Here's how the part is built. I have some questions about the finished solid (model axes, mm). Face numbers are marked on the shaded views. A direction names the side the tool comes from. Round coordinates to 2 decimals unless told otherwise and drop trailing zeros. Order: outer loops, then holes, each group sorted by start corner. A loop starts at its lowest first (then second) coordinate and runs counter-clockwise, first axis right, second up. Notation, with made-up numbers: (84, 31.25) - (113, 31.25) arc R19 cw to (113, 51.25) - close; hole circle Ø5 at (8, 25). An arc over 180 degrees is marked (long way). One line per item, written item: value.
from build123d import *

# Parameters (mm, degrees)
SCALE1_SCALE = 1.70603675


with BuildPart() as part:
    # Esquisse1 → Révolution1 (revolve)
    with BuildSketch(Plane.XY, mode=Mode.PRIVATE) as r_volution1_sk:
        with BuildLine():
            Line((1.981656821, 8.97797736), (7.823456821, 8.97797736))
            Line((7.823456821, 8.97797736), (4.683813218, 2.298439639))
            ThreePointArc((4.683813218, 2.298439639), (3.207806254, 0.623149289), (1.06377284, 0))
            Line((1.06377284, 0), (0.803456821, 0))
            Line((0.803456821, 0), (-5.036543179, 0))
            Line((-5.036543179, 0), (-15.076543179, 1.81597736))
            Line((-15.076543179, 1.81597736), (-15.076543179, 4.15197736))
            Line((-15.076543179, 4.15197736), (-2.000513414, 4.15197736))
            ThreePointArc((-2.000513414, 4.15197736), (-1.65849327, 4.212284739), (-1.357725804, 4.385932917))
            Line((-1.357725804, 4.385932917), (-0.12815557, 5.417664847))
            ThreePointArc((-0.12815557, 5.417664847), (0.135364608, 5.761091028), (0.229056821, 6.18370929))
            Line((0.229056821, 6.18370929), (0.229056821, 7.34597736))
            Line((0.229056821, 7.34597736), (1.981656821, 7.34597736))
            Line((1.981656821, 7.34597736), (1.981656821, 8.97797736))
        make_face()
    revolve(r_volution1_sk.sketch.rotate(Axis((-19.476947674, -3.82202264, 0), (1, 0, 0)), 90), axis=Axis((-19.476947674, -3.82202264, 0), (1, 0, 0)))


with BuildPart() as part_1:
    # Scale1: scaled about (-1.246951402, -3.82202264, 0)
    add(part.part.scale(SCALE1_SCALE).moved(Location((0.880393515, 2.698488443, 0))))


solid = part_1.part
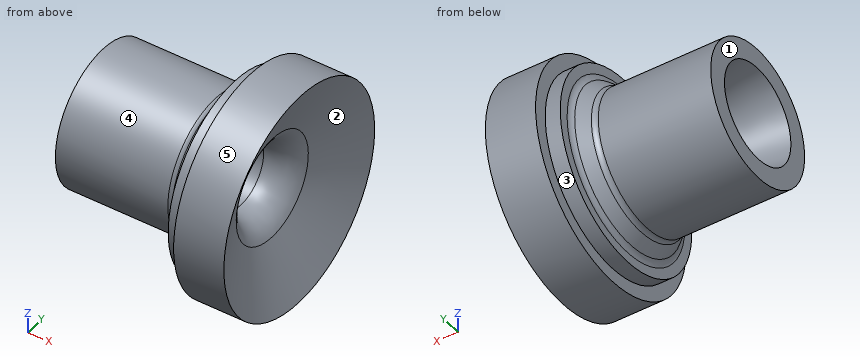
Q1. Which directions (+Z, -Z, +X, -X, +Y, -Y) give clear straight access to the entire face, cutting with the end or side of a thin tool? Please do the marked faces 4 and 5.
Results list:
face 4: -X
face 5: +X, -X
Q2. Will these pins go through, and if not, where does the flat tip stop? pin 1 (8 mm diameter, centred on x = -16.5, z = 13.5, fed in from +Y); pin 2 (3 mm diameter, centred on x = -13.5, z = 2.5, fed in from -Y); pin 3 (3 mm diameter, centred on x = 6.5, z = -3.5, fed in from +Y).
Results list:
pin 1: y = 5.92
pin 2: y = -17.39
pin 3: y = 17.92
Q3. We'd pull the mould along Y, two halves only. Please class the marked faces 1, 2 and 3: released by +Y, released by -Y, zero draft, split by the parting line, or undercut.
Results list:
face 1: zero draft
face 2: undercut
face 3: split by the parting line
Q4. If we section it at A-A, the plane z = 0: Please give me the cut outline in (x, y), then the cut area to 3 significant figures.
Results list:
outline: (-24.84, -17.43) - (-2.53, -17.43) arc R1.71 cw to (-1.44, -17.83) - (0.66, -19.59) arc R1.71 cw to (1.27, -20.89) - (1.27, -22.88) - (4.26, -22.88) - (4.26, -25.66) - (14.23, -25.66) - (8.87, -14.26) arc R6.82 ccw to (2.7, -10.34) - (-7.71, -10.34) - (-24.84, -13.44) - close; (-24.84, 5.8) - (-7.71, 2.7) - (2.7, 2.7) arc R6.82 ccw to (8.87, 6.62) - (14.23, 18.02) - (4.26, 18.02) - (4.26, 15.23) - (1.27, 15.23) - (1.27, 13.25) arc R1.71 cw to (0.66, 11.94) - (-1.44, 10.18) arc R1.71 cw to (-2.53, 9.78) - (-24.84, 9.78) - close
area: 589 mm²
Q5. If I drill on line 1 along Z through (x, y) = (9, -1); line 2 along Z through (x, y) = (-4, -1); line 3 along Y through (x, z) = (12.5, 8), over which ranges is the centre line in solid material (lowest first)?
Results list:
line 1: -21.65 to -10.34, 10.34 to 21.65
line 2: -13.31 to -5.88, 5.88 to 13.31
line 3: -24.14 to -20.13, 12.48 to 16.5
Q6. If we section it at B-B, the plane x = 0: Please give me the cut outline in (y, z), then the cut area to 3 significant figures.
Results list:
outline: circle Ø30.42 at (-3.82, 0); hole circle Ø13.04 at (-3.82, 0)
area: 593 mm²
